Here's how the part is built. I have some questions about the finished solid (model axes, mm). A direction names the side the tool comes from. Give positions to 0.01 mm unless a question says otherwise; leave off trailing zeros. Write each loop counter-clockwise with the first axis right and the second up, starting at its lowest first coordinate (ties: lowest second). Pieces come first, ordered by that corner, then holes. Notation, with made-up numbers: (45.5, 60) -> (94.5, 60) arc R25 cw to (94.5, 86) -> close; hole circle Ø1 at (33, -27). An arc over 180 degrees is marked (long way). Return JSON: item names as keys, results as strings.
from build123d import *

# Parameters (mm, degrees)
F1_DEPTH  = 38
F0_W      = 25
F0_H      = 10
F3_DEPTH  = 5
F4_DEPTH  = 10
F5_DEPTH  = 15
F6_DEPTH  = 20
F7_DEPTH  = 25
F0_W_2    = 10
F0_H_2    = 23
F8_DEPTH  = 25
F9_DEPTH  = 30
F10_DEPTH = 35
F0_W_3    = 5
F0_H_3    = 28
F11_DEPTH = 38
F12_DEPTH = 15


# Not quite as in the source:
# - a feature names something its author has since deleted; it is built from what else it names


with BuildPart() as f1:
    # F0 (on Top) → F1 (new body)
    with BuildSketch(Plane.XY):
        Polygon((-33.5, 19), (-38.5, 19), (-38.5, -24), (-33.5, -24), (-33.5, -14), (-33.5, -4), align=None)
        Polygon((11.5, 24), (-38.5, 24), (-38.5, 19), (-33.5, 19), (-8.5, 19), (1.5, 19), (11.5, 19), align=None)
    extrude(amount=F1_DEPTH)

    # F0 (on Top) → F3 (join)
    with BuildSketch(Plane.XY):
        with Locations((-21, -19)):
            Rectangle(F0_W, F0_H)
    extrude(amount=F3_DEPTH)

    # F0 (on Top) → F4 (join)
    with BuildSketch(Plane.XY):
        Polygon((33.5, -14), (33.5, -4), (11.5, -4), (1.5, -4), (-8.5, -4), (-33.5, -4), (-33.5, -14), (-8.5, -14), align=None)
    extrude(amount=F4_DEPTH)

    # F0 (on Top) → F5 (join)
    with BuildSketch(Plane.XY):
        Polygon((-8.5, -4), (-33.5, 19), (-33.5, -4), align=None)
    extrude(amount=F5_DEPTH)

    # F0 (on Top) → F6 (join)
    with BuildSketch(Plane.XY):
        Polygon((-8.5, 19), (-33.5, 19), (-8.5, -4), align=None)
    extrude(amount=F6_DEPTH)

    # F2 (on face) → F7 (cut)
    with BuildSketch(Plane.YZ.offset(-33.5)):
        Polygon((-24, 14), (19, 38), (-24, 38), align=None)
    extrude(amount=-F7_DEPTH, mode=Mode.SUBTRACT)

    # F0 (on Top) → F8 (join)
    with BuildSketch(Plane.XY):
        with Locations((-3.5, 7.5)):
            Rectangle(F0_W_2, F0_H_2)
    extrude(amount=F8_DEPTH)

    # F0 (on Top) → F9 (join)
    with BuildSketch(Plane.XY):
        with Locations((6.5, 7.5)):
            Rectangle(F0_W_2, F0_H_2)
    extrude(amount=F9_DEPTH)

    # F0 (on Top) → F10 (join)
    with BuildSketch(Plane.XY):
        Polygon((33.5, 24), (11.5, 24), (11.5, 19), (11.5, -4), (33.5, -4), align=None)
    extrude(amount=F10_DEPTH)

    # F0 (on Top) → F11 (join)
    with BuildSketch(Plane.XY):
        with Locations((36, 10)):
            Rectangle(F0_W_3, F0_H_3)
    extrude(amount=F11_DEPTH)

    # F0 (on Top) → F12 (join)
    with BuildSketch(Plane.XY):
        Polygon((38.5, -4), (33.5, -4), (33.5, -14), (33.5, -24), (38.5, -24), align=None)
    extrude(amount=F12_DEPTH)


solid = f1.part
1. If we mould it in two halves opening along X, with no side actions, what happens to faces 6 (the face through (7, -14, 5)), 7 (the face through (-1, 24, 19)), 8 (the face through (-27, 3, 15))? For each: released by +X, released by -X, zero draft, split by the parting line, or undercut.
Taken from the geometry:
{"face 6": "undercut", "face 7": "zero draft", "face 8": "undercut"}
2. If I drill on line 1 (X direction, y = 18, z = 22.5); line 2 (X direction, y = 8.5, z = 27); line 3 (Z direction, x = -15.5, y = -20), over which ranges is the centre line in solid material (lowest first)? Write a range as [from, to].
Taken from the geometry:
{"line 1": "x = [-38.5, -33.5], [-8.5, 38.5]", "line 2": "x = [-38.5, -33.5], [1.5, 38.5]", "line 3": "z = [0, 5]"}
3. Suppose I cut it at D-D, the plane y = 1.5. List the corners of the cut face in (x, z) for me, and give its area (3 significant figures).
Taken from the geometry:
{"outline": "(-38.5, 0) -> (38.5, 0) -> (38.5, 38) -> (33.5, 38) -> (33.5, 35) -> (11.5, 35) -> (11.5, 30) -> (1.5, 30) -> (1.5, 25) -> (-8.5, 25) -> (-8.5, 20) -> (-14.48, 20) -> (-14.48, 15) -> (-33.5, 15) -> (-33.5, 28.23) -> (-38.5, 28.23) -> close", "area": "2,060 mm²"}
4. Suppose I cut it at C-C, the plane y = -16.5. List the corners of the cut face in (x, z) for me.
Taken from the geometry:
{"outline": "(-38.5, 0) -> (-8.5, 0) -> (-8.5, 5) -> (-33.5, 5) -> (-33.5, 18.19) -> (-38.5, 18.19) -> close; (33.5, 0) -> (38.5, 0) -> (38.5, 15) -> (33.5, 15) -> close"}
5. Suppose I cut it at A-A, the plane z = 12. List the corners of the cut face in (x, y) for me.
Taken from the geometry:
{"outline": "(-38.5, -24) -> (-33.5, -24) -> (-33.5, -4) -> (33.5, -4) -> (33.5, -24) -> (38.5, -24) -> (38.5, 24) -> (-38.5, 24) -> close"}
6. Which directions (+Z, -Z, +X, -X, +Y, -Y) give clear straight access to the entire face, cutting with the end or side of a thin tool? Please do faces 1 (the face through (22, 10, 35)), 2 (the face through (36, 10, 38)), 3 (the face through (-1, 0, 0)), 4 (the face through (33.5, -16, 9)), 5 (the face through (36, -14, 15)).
Taken from the geometry:
{"face 1": "+Z, +Y, -Y", "face 2": "+Z, +X, -X, +Y, -Y", "face 3": "-Z, +X, -X, +Y, -Y", "face 4": "+Z, -Y", "face 5": "+Z, +X, -Y"}
7. Suppose I cut it at B-B, the plane x = -3. List the corners of the cut face in (y, z) for me.
Taken from the geometry:
{"outline": "(-14, 0) -> (24, 0) -> (24, 38) -> (19, 38) -> (19, 25) -> (-4, 25) -> (-4, 10) -> (-14, 10) -> close"}
8. For pin 1 Ø9 at (x, z) = (-19, 25.5) entering from -Y; pin 2 Ø2.5 at (y, z) = (5.5, 36.5) entering from -X; pin 3 Ø3 at (x, y) = (-27.5, 1) entering from +Z; pin 4 Ø1.5 at (y, z) = (-13.5, 21.5) entering from -X, each with a flat end and sliding along its axis, tell me the tip position at first contact or that it passes through.
Taken from the geometry:
{"pin 1": "stops at y = 19", "pin 2": "stops at x = 33.5", "pin 3": "stops at z = 15", "pin 4": "passes through"}
